```python
from build123d import *

# Parameters (mm, degrees)
CUT_EXTRUDE1_DEPTH = 20
SKETCH5_R          = 3.5
CUT_EXTRUDE2_DEPTH = 50


with BuildPart() as part:
    # Sketch2 → Revolve1 (revolve)
    with BuildSketch(Plane.XY, mode=Mode.PRIVATE) as revolve1_sk:
        Polygon((0, 0), (0, 10), (43, 10), (45, 8), (75, 8), (77, 10), (120, 10), (120, 4), (120, 0), align=None)
    revolve(revolve1_sk.sketch.rotate(Axis((120, 0, 0), (-1, 0, 0)), 90), axis=Axis((120, 0, 0), (-1, 0, 0)))

    # Sketch3 → Cut-Extrude1 (cut)
    with BuildSketch(Plane.ZY):
        with BuildLine():
            Line((-1.183215957, 1.15), (1.183215957, 1.15))
            ThreePointArc((1.183215957, 1.15), (0, -1.65), (-1.183215957, 1.15))
        make_face()
    extrude(amount=-CUT_EXTRUDE1_DEPTH, mode=Mode.SUBTRACT)

    # Sketch5 → Cut-Extrude2 (cut)
    with BuildSketch(Plane(origin=(120, 0, 0), x_dir=(0, 0, -1), z_dir=(1, 0, 0))):
        Circle(SKETCH5_R)
    extrude(amount=-CUT_EXTRUDE2_DEPTH, mode=Mode.SUBTRACT)


solid = part.part
```
Model file for the job. Use its own axes, mm. A direction names the side the tool comes from. Coordinates: 2 decimals unless noted, no trailing zeros. Order: outer loops, then holes, each group sorted by start corner. A loop starts at its lowest first (then second) coordinate and runs counter-clockwise, first axis right, second up. Notation, with made-up numbers: (45.25, 31) -> (60.25, 31) arc R9 cw to (60.25, 42) -> close; hole circle Ø4 at (89, 35). An arc over 180 degrees is marked (long way). Return JSON: item names as keys, results as strings.
Item 1: Mould opens along Y. For faces 1 (the face through (120, 0, 4)), 2 (the face through (10, 1.15, 0)), 3 (the face through (22, 0, 10)) say: pulls with the +Y half, pulls with the -Y half, needs draft (parallel to the pull), parting line crosses it, or undercut.
Model answer:
{"face 1": "needs draft", "face 2": "undercut", "face 3": "parting line crosses it"}
Item 2: Slice it at C-C (x = 46). Write the cut outline in (y, z).
Model answer:
{"outline": "circle Ø16 at (0, 0)"}
Item 3: Slice it at A-A (y = 0). Write the cut outline in (x, z), then the cut area to 3 significant figures.
Model answer:
{"outline": "(0, -10) -> (43, -10) -> (45, -8) -> (75, -8) -> (77, -10) -> (120, -10) -> (120, -3.5) -> (70, -3.5) -> (70, 3.5) -> (120, 3.5) -> (120, 10) -> (77, 10) -> (75, 8) -> (45, 8) -> (43, 10) -> (0, 10) -> (0, 1.65) -> (20, 1.65) -> (20, -1.65) -> (0, -1.65) -> close", "area": "1,860 mm²"}
Item 4: Slice it at D-D (x = 12). Write the cut outline in (y, z).
Model answer:
{"outline": "circle Ø20 at (0, 0); hole (1.15, -1.18) -> (1.15, 1.18) arc R1.65 ccw (long way) to start"}
Item 5: Pin check, flat tips, straight feed: P1, Ø4.5, axis at y = 0, z = 0, coming from the +X side; P2, Ø12, axis at y = 3.5, z = 7, coming from the -X side; P3, Ø8, axis at x = 16, y = -4.5, coming from the +Z side; P4, Ø2, axis at y = 0, z = 0.5, coming from the -X side. Stop position of each tip, or through.
Model answer:
{"P1": "stops at x = 70", "P2": "stops at x = 0", "P3": "stops at z = 9.99", "P4": "stops at x = 20"}
Item 6: 3-axis set-ups, long thin cutter, end or side, ignore diameter. For faces 4 (the face through (75.125, -2.441, -7.75)), 5 (the face through (95.35, -1.341, -3.233)), 6 (the face through (9.86, -1.65, 0.05)), 7 (the face through (99, 0, 10)): which of +Z, -Z, +X, -X, +Y, -Y reach the whole face in a straight line?
Model answer:
{"face 4": "none", "face 5": "+X", "face 6": "-X", "face 7": "+X, -X"}
Item 7: Wall check: line 1 along Y through (x, z) = (87.5, 0); line 2 along Y through (x, z) = (12.25, 0); line 3 along Y through (x, z) = (48.5, -0.25). Give the ranges that are in metal, low to high. Write a range as from..to.
Model answer:
{"line 1": "y = -10..-3.5, 3.5..10", "line 2": "y = -10..-1.65, 1.15..10", "line 3": "y = -8..8"}
Item 8: Slice it at B-B (z = 0). Write the cut outline in (x, y), then the cut area to 3 significant figures.
Model answer:
{"outline": "(0, -10) -> (43, -10) -> (45, -8) -> (75, -8) -> (77, -10) -> (120, -10) -> (120, -3.5) -> (70, -3.5) -> (70, 3.5) -> (120, 3.5) -> (120, 10) -> (77, 10) -> (75, 8) -> (45, 8) -> (43, 10) -> (0, 10) -> (0, 1.15) -> (20, 1.15) -> (20, -1.65) -> (0, -1.65) -> close", "area": "1,870 mm²"}
